Work out the finished part from the listing and answer in its coordinate system (mm). Give positions to 0.01 mm unless a question says otherwise; leave off trailing zeros. Write each loop counter-clockwise with the first axis right and the second up, starting at its lowest first coordinate (ties: lowest second). Pieces come first, ordered by that corner, then holes. Notation, with made-up numbers: (-18.5, -39) - (-0.5, -39) arc R4 cw to (-0.5, -32) - close; hole circle Ø8 at (63, 42.25). An arc over 180 degrees is marked (long way). Write item = value, one per line.
from build123d import *

# Parameters (mm, degrees)
SKETCH1_R           = 2.4384
BOSS_EXTRUDE1_DEPTH = 3.175
CUT_EXTRUDE1_START  = -3.048
SKETCH2_R           = 2.4384
CUT_EXTRUDE1_DEPTH  = 3.048
CUT_EXTRUDE2_START  = -3.048
SKETCH3_R           = 2.4384
CUT_EXTRUDE2_DEPTH  = 3.048
SKETCH7_R           = 2.5019
CUT_EXTRUDE6_DEPTH  = 249.108397571
CUT_EXTRUDE7_DEPTH  = 3.175
FILLET1_R           = 25.4
FILLET2_R           = 1.27
FILLET5_R           = 5.08


with BuildPart() as part:
    # Sketch1 → Boss-Extrude1 (new body)
    with BuildSketch(Plane(origin=(0, 0, 0), x_dir=(0, 0, -1), z_dir=(1, 0, 0))):
        with BuildLine():
            ThreePointArc((223.742915845, -76.264038282), (234.613620352, -73.464824815), (231.814406885, -62.594120308))
            Line((231.814406885, -62.594120308), (163.445060929, -22.225))
            Line((163.445060929, -22.225), (160.3375, -22.225))
            Line((160.3375, -22.225), (160.3375, -19.05))
            Line((160.3375, -19.05), (147.6375, -19.05))
            Line((147.6375, -19.05), (147.6375, -22.225))
            Line((147.6375, -22.225), (134.9375, -22.225))
            Line((134.9375, -22.225), (134.9375, -19.05))
            Line((134.9375, -19.05), (122.2375, -19.05))
            Line((122.2375, -19.05), (122.2375, -22.225))
            Line((122.2375, -22.225), (109.5375, -22.225))
            Line((109.5375, -22.225), (109.5375, -19.05))
            Line((109.5375, -19.05), (96.8375, -19.05))
            Line((96.8375, -19.05), (96.8375, -22.225))
            Line((96.8375, -22.225), (84.1375, -22.225))
            Line((84.1375, -22.225), (84.1375, -19.05))
            Line((84.1375, -19.05), (71.4375, -19.05))
            Line((71.4375, -19.05), (71.4375, -22.225))
            Line((71.4375, -22.225), (58.7375, -22.225))
            Line((58.7375, -22.225), (58.7375, -19.05))
            Line((58.7375, -19.05), (46.0375, -19.05))
            Line((46.0375, -19.05), (46.0375, -22.225))
            Line((46.0375, -22.225), (33.3375, -22.225))
            Line((33.3375, -22.225), (33.3375, -19.05))
            Line((33.3375, -19.05), (20.6375, -19.05))
            Line((20.6375, -19.05), (20.6375, -22.225))
            Line((20.6375, -22.225), (7.9375, -22.225))
            Line((7.9375, -22.225), (7.9375, 0))
            ThreePointArc((7.9375, 0), (-4.92125, 12.85875), (-17.78, 0))
            Line((-17.78, 0), (-17.78, -31.4325))
            ThreePointArc((-17.78, -31.4325), (-14.897198494, -38.392198494), (-7.9375, -41.275))
            Line((-7.9375, -41.275), (4.7625, -41.275))
            Line((4.7625, -41.275), (4.7625, -44.45))
            Line((4.7625, -44.45), (17.4625, -44.45))
            Line((17.4625, -44.45), (17.4625, -41.275))
            Line((17.4625, -41.275), (30.1625, -41.275))
            Line((30.1625, -41.275), (30.1625, -44.45))
            Line((30.1625, -44.45), (42.8625, -44.45))
            Line((42.8625, -44.45), (42.8625, -41.275))
            Line((42.8625, -41.275), (55.5625, -41.275))
            Line((55.5625, -41.275), (55.5625, -44.45))
            Line((55.5625, -44.45), (68.2625, -44.45))
            Line((68.2625, -44.45), (68.2625, -41.275))
            Line((68.2625, -41.275), (80.9625, -41.275))
            Line((80.9625, -41.275), (80.9625, -44.45))
            Line((80.9625, -44.45), (93.6625, -44.45))
            Line((93.6625, -44.45), (93.6625, -41.275))
            Line((93.6625, -41.275), (106.3625, -41.275))
            Line((106.3625, -41.275), (106.3625, -44.45))
            Line((106.3625, -44.45), (119.0625, -44.45))
            Line((119.0625, -44.45), (119.0625, -41.275))
            Line((119.0625, -41.275), (131.7625, -41.275))
            Line((131.7625, -41.275), (131.7625, -44.45))
            Line((131.7625, -44.45), (144.4625, -44.45))
            Line((144.4625, -44.45), (144.4625, -41.275))
            Line((144.4625, -41.275), (157.1625, -41.275))
            Line((157.1625, -41.275), (157.1625, -44.45))
            Line((157.1625, -44.45), (169.8625, -44.45))
            Line((169.8625, -44.45), (223.742915845, -76.264038282))
        make_face()
        with Locations((227.778661365, -69.429079295)):
            Circle(SKETCH1_R, mode=Mode.SUBTRACT)
        Circle(SKETCH1_R, mode=Mode.SUBTRACT)
    extrude(amount=BOSS_EXTRUDE1_DEPTH)

    # Sketch2 → Cut-Extrude1 (cut)
    with BuildSketch(Plane(origin=(3.175, 0, 0), x_dir=(0, 0, -1), z_dir=(1, 0, 0)).offset(CUT_EXTRUDE1_START)):
        Polygon((2.419674978, 4.191), (-2.419674978, 4.191), (-4.839349956, 0), (-2.419674978, -4.191), (2.419674978, -4.191), (4.839349956, 0), align=None)
        Circle(SKETCH2_R, mode=Mode.SUBTRACT)
    extrude(amount=CUT_EXTRUDE1_DEPTH, mode=Mode.SUBTRACT)

    # Sketch3 → Cut-Extrude2 (cut)
    with BuildSketch(Plane(origin=(3.175, 0, 0), x_dir=(0, 0, -1), z_dir=(1, 0, 0)).offset(CUT_EXTRUDE2_START)):
        Polygon((230.198336343, -65.238079295), (225.358986387, -65.238079295), (222.939311409, -69.429079295), (225.358986387, -73.620079295), (230.198336343, -73.620079295), (232.618011321, -69.429079295), align=None)
        with Locations((227.778661365, -69.429079295)):
            Circle(SKETCH3_R, mode=Mode.SUBTRACT)
    extrude(amount=CUT_EXTRUDE2_DEPTH, mode=Mode.SUBTRACT)

    # Sketch7 → Cut-Extrude6 (cut, through all)
    with BuildSketch(Plane.ZY):
        with Locations((-201.805817216, -54.09324632)):
            Circle(SKETCH7_R)
        with Locations((-179.933948459, -41.178860656)):
            Circle(SKETCH7_R)
    extrude(amount=-CUT_EXTRUDE6_DEPTH, mode=Mode.SUBTRACT)

    # Sketch9 → Cut-Extrude7 (cut)
    with BuildSketch(Plane(origin=(3.175, 0, 0), x_dir=(0, 0, -1), z_dir=(1, 0, 0))):
        with BuildLine():
            Line((58.74893, -28.575), (63.69939, -28.575))
            ThreePointArc((63.69939, -28.575), (66.87439, -31.75), (63.69939, -34.925))
            Line((63.69939, -34.925), (58.74893, -34.925))
            ThreePointArc((58.74893, -34.925), (55.57393, -31.75), (58.74893, -28.575))
        make_face()
        with BuildLine():
            Line((154.37485, -28.575), (149.42439, -28.575))
            ThreePointArc((149.42439, -28.575), (146.24939, -31.75), (149.42439, -34.925))
            Line((149.42439, -34.925), (154.37485, -34.925))
            ThreePointArc((154.37485, -34.925), (157.54985, -31.75), (154.37485, -28.575))
        make_face()
    extrude(amount=-CUT_EXTRUDE7_DEPTH, mode=Mode.SUBTRACT)

    # Fillet1
    fillet1_edges = [part.edges().sort_by_distance(p)[0] for p in [
        (1.5875, -44.45, -169.8625),
    ]]
    fillet(fillet1_edges, radius=FILLET1_R)

    # Fillet2
    fillet2_edges = [part.edges().sort_by_distance(p)[0] for p in [
        (1.5875, -22.225, -7.9375),
    ]]
    fillet(fillet2_edges, radius=FILLET2_R)

    # Fillet5
    fillet5_edges = [part.edges().sort_by_distance(p)[0] for p in [
        (1.5875, -22.225, -163.445060929),
    ]]
    fillet(fillet5_edges, radius=FILLET5_R)


solid = part.part
1. Find section A-A, the plane z = 0. Give the vertices of the cut face in (x, y) (3 decimals).
Solution:
outline = (0, -41.275) - (3.175, -41.275) - (3.175, -4.191) - (0.127, -4.191) - (0.127, -2.438) - (0, -2.438) - close; (0, 2.438) - (0.127, 2.438) - (0.127, 4.191) - (3.175, 4.191) - (3.175, 11.88) - (0, 11.88) - close
2. Given pin 1 (1.5 mm diameter, centred on x = 2, z = 0.5, fed in from -Y) (3 decimals); pin 2 (1 mm diameter, centred on x = 1.5, z = -115, fed in from -Y); pin 3 (1 mm diameter, centred on x = 1.5, z = -35.5, fed in from +Y) (3 decimals); pin 4 (1 mm diameter, centred on y = -21.5, z = -112, fed in from -X), each flat-ended and moving along its own axis, determine where each tip first touches the part or whether it passes through.
Solution:
pin_1 = -41.275
pin_2 = -44.45
pin_3 = -22.225
pin_4 = through
3. Find section B-B, the plane x = 1.6. Give the number of separate pieces and of enclosed holes in the cut face, then the cut area to 3 significant figures.
Solution:
separate_pieces = 1
enclosed_holes = 6
area = 5,780 mm^2
4. Straight lines are drawn through the part: line 1 (Z direction, x = 1.35, y = -30); line 2 (Z direction, x = 0.85, y = -34.5); line 3 (Z direction, x = 1.5, y = -8.5). For each, find the intervals that lie inside material, in ascending order.
Solution:
line_1 = -176.61 to -157.02, -146.78 to -66.35, -56.1 to 17.78
line_2 = -184.23 to -155.96, -147.84 to -65.29, -57.16 to 17.29
line_3 = -7.94 to 17.78
5. For a pull along Z with two mould halves and no side action, classify faces 1 (the cylindrical face through (1.565, -53.983, -204.305)), 2 (the flat face through (1.57, -43.04, -198.7)), 3 (the cylindrical face through (1.565, -41.069, -182.433)), 4 (the flat face through (0, -32, -90)) as pulls with the +Z half, pulls with the -Z half, needs draft (parallel to the pull), parting line crosses it, or undercut.
Solution:
face_1 = undercut
face_2 = pulls with the -Z half
face_3 = undercut
face_4 = needs draft
